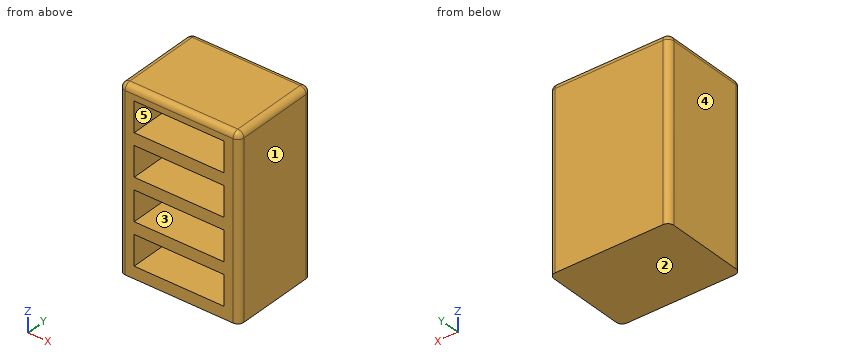
from build123d import *

# Parameters (mm, degrees)
F0_W     = 101.6
F0_H     = 76.2
F1_DEPTH = 152.4
F2_W     = 76.2
F2_H     = 25.4
F3_DEPTH = 55.88
F4_R     = 5.08


with BuildPart() as f1:
    # F0 (on Top) → F1 (new body)
    with BuildSketch(Plane.XY):
        Rectangle(F0_W, F0_H)
    extrude(amount=F1_DEPTH)

    # F2 (on face) → F3 (cut)
    with BuildSketch(Plane.XZ.offset(38.1)):
        with Locations((0, 129.54)):
            Rectangle(F2_W, F2_H)
        with Locations((0, 93.98)):
            Rectangle(F2_W, F2_H)
        with Locations((0, 58.42)):
            Rectangle(F2_W, F2_H)
        with Locations((0, 22.86)):
            Rectangle(F2_W, F2_H)
    extrude(amount=-F3_DEPTH, mode=Mode.SUBTRACT)

    # F4
    f4_edges = [f1.edges().sort_by_distance(p)[0] for p in [
        (50.8, 0, 152.4),
        (-50.8, 0, 152.4),
        (0, -38.1, 152.4),
        (0, 38.1, 152.4),
        (50.8, -38.1, 76.2),
        (50.8, 38.1, 76.2),
        (-50.8, -38.1, 76.2),
        (-50.8, 38.1, 76.2),
    ]]
    fillet(f4_edges, radius=F4_R)


solid = f1.part
Read the model definition and answer for the solid it produces. Units are mm, in the model's axes. Face numbers are marked on the shaded views. A direction names the side the tool comes from. Give positions to 0.01 mm unless a question says otherwise; leave off trailing zeros. Write each loop counter-clockwise with the first axis right and the second up, starting at its lowest first coordinate (ties: lowest second). Pieces come first, ordered by that corner, then holes. Notation, with made-up numbers: (-24.75, 6) - (1.25, 6) arc R18 cw to (1.25, 22) - close; hole circle Ø8 at (-22, 55). An arc over 180 degrees is marked (long way). Return JSON: item names as keys, results as strings.
Q1. Given P1, Ø17, axis at x = -1, y = -4, coming from the -Z side; P2, Ø20.5, axis at x = 9, z = 93.5, coming from the -Y side, each flat-ended and moving along its own axis, determine where each tip first touches the part or whether it passes through.
Reply:
{"P1": "z = 0", "P2": "y = 17.78"}
Q2. A cutting plane is placed at B-B, the plane z = 30. Determine the outline of the cut face in (x, y), and give its area (3 significant figures).
Reply:
{"outline": "(-50.8, -33.02) arc R5.08 ccw to (-45.72, -38.1) - (-38.1, -38.1) - (-38.1, 17.78) - (38.1, 17.78) - (38.1, -38.1) - (45.72, -38.1) arc R5.08 ccw to (50.8, -33.02) - (50.8, 33.02) arc R5.08 ccw to (45.72, 38.1) - (-45.72, 38.1) arc R5.08 ccw to (-50.8, 33.02) - close", "area": "3,460 mm²"}
Q3. For a pull along X with two mould halves and no side action, classify the marked faces 1, 2 and 3 as released by +X, released by -X, zero draft, split by the parting line, or undercut.
Reply:
{"face 1": "released by +X", "face 2": "zero draft", "face 3": "undercut"}
Q4. A cutting plane is placed at A-A, the plane y = 12. Determine the outline of the cut face in (x, z), and give its area (3 significant figures).
Reply:
{"outline": "(-50.8, 0) - (50.8, 0) - (50.8, 147.32) arc R5.08 ccw to (45.72, 152.4) - (-45.72, 152.4) arc R5.08 ccw to (-50.8, 147.32) - close; hole (-38.1, 10.16) - (38.1, 10.16) - (38.1, 35.56) - (-38.1, 35.56) - close; hole (-38.1, 45.72) - (38.1, 45.72) - (38.1, 71.12) - (-38.1, 71.12) - close; hole (-38.1, 81.28) - (38.1, 81.28) - (38.1, 106.68) - (-38.1, 106.68) - close; hole (-38.1, 116.84) - (38.1, 116.84) - (38.1, 142.24) - (-38.1, 142.24) - close", "area": "7,730 mm²"}
Q5. Consider line 1 along Z through (x, y) = (37, 8); line 2 along X through (y, z) = (-25, 125); line 3 along Y through (x, z) = (-10, 82). Determine where each line is inside the solid, lowest interval first. Write a range as [from, to].
Reply:
{"line 1": "[0, 10.16], [35.56, 45.72], [71.12, 81.28], [106.68, 116.84], [142.24, 152.4]", "line 2": "[-50.8, -38.1], [38.1, 50.8]", "line 3": "[17.78, 38.1]"}
Q6. For the marked faces 4 and 5, determine the directions among +Z, -Z, +X, -X, +Y, -Y from which every point of the face is accessible in a straight line to the end or side of a thin tool.
Reply:
{"face 4": "+Z, -Z, -X, +Y, -Y", "face 5": "-Y"}
Q7. A cutting plane is placed at C-C, the plane x = -31.5. Determine the outline of the cut face in (y, z), and give its area (3 significant figures).
Reply:
{"outline": "(-38.1, 0) - (38.1, 0) - (38.1, 147.32) arc R5.08 ccw to (33.02, 152.4) - (-33.02, 152.4) arc R5.08 ccw to (-38.1, 147.32) - (-38.1, 142.24) - (17.78, 142.24) - (17.78, 116.84) - (-38.1, 116.84) - (-38.1, 106.68) - (17.78, 106.68) - (17.78, 81.28) - (-38.1, 81.28) - (-38.1, 71.12) - (17.78, 71.12) - (17.78, 45.72) - (-38.1, 45.72) - (-38.1, 35.56) - (17.78, 35.56) - (17.78, 10.16) - (-38.1, 10.16) - close", "area": "5,920 mm²"}
